Geometry: final body of the model. Coordinates: model frame, mm. Round coordinates to 2 decimals unless told otherwise and drop trailing zeros. Loops run counter-clockwise (first coordinate to the right, second up) from the corner with the lowest first, then second, coordinate; pieces in that order, holes last. Notation, with made-up numbers: (79.25, -28) - (84.25, -28) arc R8 ccw to (84.25, -14) - close; hole circle Ø4 at (37.5, -15.5). An arc over 180 degrees is marked (long way). Return JSON: item names as keys, results as strings. Group by question number.
1. Section B-B on z = 3.55. Return loops of the section in (x, y).
2. Section C-C on y = -25. Return loops of the section in (x, z), and give its area (3 significant figures).
3. Section D-D on x = 0. Return loops of the section in (y, z), and give its area (3 significant figures).
4. Draft query along Y for faces 1 (the face through (-59.85, 0, 2)), 2 (the face through (-19.956, -29.752, 2.465)), 3 (the face through (18.65, 28.57, 2.54)), 4 (the face through (13.444, 23.692, 2.535)). Return one class per face: +Y half, -Y half, draft (parallel to the pull), parting line (faces both ways), or undercut.
5. Section A-A on x = -34.85. Return loops of the section in (y, z), and give its area (3 significant figures).
6. Material intervals for probe 1 along Y at (x, z) = (-54.85, 2.95); probe 2 along X at (y, z) = (-9, 2); probe 3 along X at (y, z) = (-10, 1.25), sorted ascending.
7. First-contact query: pin 1 Ø7 at (x, y) = (15.15, 25) entering from +Z; pin 2 Ø1.5 at (y, z) = (-2, 2) entering from +X. Flat tips, straight axial feed; report the tip coordinate or a pass-through.
from build123d import *

# Parameters (mm, degrees)
SKETCH_1_W          = 80
SKETCH_1_H          = 60
SKETCH_1_R          = 7.65
EXTRUDE_1_DEPTH     = 5
SKETCH_2_R          = 2.15
CUT_EXTRUDE_1_DEPTH = 68.134361545
SKETCH_3_R          = 2.15
CUT_EXTRUDE_2_DEPTH = 68.134361545
CUT_EXTRUDE_3_DEPTH = 68.134361545
SKETCH_6_R          = 2.15
CUT_EXTRUDE_5_DEPTH = 68.134361545
FILLET_1_R          = 5


with BuildPart() as part:
    # ｽｹｯﾁ1 → ﾎﾞｽ - 押し出し1 (new body)
    with BuildSketch(Plane.XY):
        with Locations((-19.85, 0)):
            Rectangle(SKETCH_1_W, SKETCH_1_H)
        with Locations((0, 10)):
            Circle(SKETCH_1_R, mode=Mode.SUBTRACT)
    extrude(amount=EXTRUDE_1_DEPTH)

    # ｽｹｯﾁ2 → ｶｯﾄ - 押し出し1 (cut, through all)
    with BuildSketch(Plane.XY.offset(5)):
        with Locations((-54.85, 10)):
            Circle(SKETCH_2_R)
        with Locations(Location((-54.85, -10, 0), (0, 0, 180))):
            Circle(SKETCH_2_R)
        with Locations((-34.85, 10)):
            Circle(SKETCH_2_R)
        with Locations(Location((-34.85, -10, 0), (0, 0, 180))):
            Circle(SKETCH_2_R)
    extrude(amount=-CUT_EXTRUDE_1_DEPTH, mode=Mode.SUBTRACT)

    # ｽｹｯﾁ3 → ｶｯﾄ - 押し出し2 (cut, through all)
    with BuildSketch(Plane.XY.offset(5)):
        with Locations((15.15, 25)):
            Circle(SKETCH_3_R)
        with BuildLine():
            ThreePointArc((15.15, 30), (18.685533906, 28.535533906), (20.15, 25))
            Line((20.15, 25), (20.15, 30))
            Line((20.15, 30), (15.15, 30))
        make_face()
    extrude(amount=-CUT_EXTRUDE_2_DEPTH, mode=Mode.SUBTRACT)

    # ｽｹｯﾁ4 → ｶｯﾄ - 押し出し3 (cut, through all)
    with BuildSketch(Plane.XY.offset(5)):
        Polygon((-59.85, 30), (-59.85, 15), (-29.85, 30), align=None)
        Polygon((-29.85, -30), (-59.85, -15), (-59.85, -30), align=None)
        with BuildLine():
            Line((20.15, 0), (17.493498792, 0))
            ThreePointArc((17.493498792, 0), (15.094907291, -3.347893986), (12.06572435, -6.138178209))
            Line((12.06572435, -6.138178209), (-19.85, -30))
            Line((-19.85, -30), (20.15, -30))
            Line((20.15, -30), (20.15, 0))
        make_face()
        with BuildLine():
            ThreePointArc((20.15, 10), (19.474553919, 4.8265824), (17.493498792, 0))
            Line((17.493498792, 0), (20.15, 0))
            Line((20.15, 0), (20.15, 10))
        make_face()
    extrude(amount=-CUT_EXTRUDE_3_DEPTH, mode=Mode.SUBTRACT)

    # ｽｹｯﾁ6 → ｶｯﾄ - 押し出し5 (cut, through all)
    with BuildSketch(Plane.XY.offset(5)):
        with Locations((-28.669660113, -25)):
            Circle(SKETCH_6_R)
    extrude(amount=-CUT_EXTRUDE_5_DEPTH, mode=Mode.SUBTRACT)

    # ﾌｨﾚｯﾄ1
    fillet_1_edges = [part.edges().sort_by_distance(p)[0] for p in [
        (-59.85, 15, 2.5),
        (-29.85, 30, 2.5),
        (-59.85, -15, 2.5),
        (-29.85, -30, 2.5),
        (-19.85, -30, 2.5),
    ]]
    fillet(fillet_1_edges, radius=FILLET_1_R)


solid = part.part
Taken from the geometry:
{
 "1": {"outline": "(-59.85, -11.91) arc R5 ccw to (-57.09, -16.38) - (-30.91, -29.47) arc R5 ccw to (-28.67, -30) - (-21.51, -30) arc R5 ccw to (-18.52, -29) - (12.07, -6.14) arc R20.15 ccw to (20.15, 10) - (20.15, 25) arc R5 ccw to (15.15, 30) - (-28.67, 30) arc R5 ccw to (-30.91, 29.47) - (-57.09, 16.38) arc R5 ccw to (-59.85, 11.91) - close; hole circle Ø4.3 at (-54.85, -10); hole circle Ø4.3 at (-54.85, 10); hole circle Ø4.3 at (-34.85, -10); hole circle Ø4.3 at (-34.85, 10); hole circle Ø4.3 at (-28.67, -25); hole circle Ø15.3 at (0, 10); hole circle Ø4.3 at (15.15, 25)"},
 "2": {"outline": "(-39.85, 0) - (-30.82, 0) - (-30.82, 5) - (-39.85, 5) - close; (-26.52, 0) - (-13.16, 0) - (-13.16, 5) - (-26.52, 5) - close", "area": "112 mm2"},
 "3": {"outline": "(-15.16, 0) - (2.35, 0) - (2.35, 5) - (-15.16, 5) - close; (17.65, 0) - (30, 0) - (30, 5) - (17.65, 5) - close", "area": "149 mm2"},
 "4": {"face 1": "draft", "face 2": "-Y half", "face 3": "+Y half", "face 4": "undercut"},
 "5": {"outline": "(-27.5, 0) - (-12.15, 0) - (-12.15, 5) - (-27.5, 5) - close; (-7.85, 0) - (7.85, 0) - (7.85, 5) - (-7.85, 5) - close; (12.15, 0) - (27.5, 0) - (27.5, 5) - (12.15, 5) - close", "area": "232 mm2"},
 "6": {"probe 1": "-17.5 to -12.15, -7.85 to 7.85, 12.15 to 17.5", "probe 2": "-59.85 to -56.75, -52.95 to -36.75, -32.95 to 8.24", "probe 3": "-59.85 to -57, -52.7 to -37, -32.7 to 6.9"},
 "7": {"pin 1": "z = 5", "pin 2": "x = 16.72"}
}
